Geometry: see drawing. Coordinates: mm, zero at the bounding-box minimum. A direction names the side the tool comes from. Coordinates: 2 decimals unless noted, no trailing zeros. Loops run counter-clockwise (first coordinate to the right, second up) from the corner with the lowest first, then second, coordinate; pieces in that order, holes last. Notation, with made-up numbers: (10, 31) - (63, 31) arc R18 cw to (63, 36) - close; hole circle Ø8 at (28, 56.25). An arc over 180 degrees is marked (long way). Write each question's results on one line, items separated by ' | '. Start each with the question number.
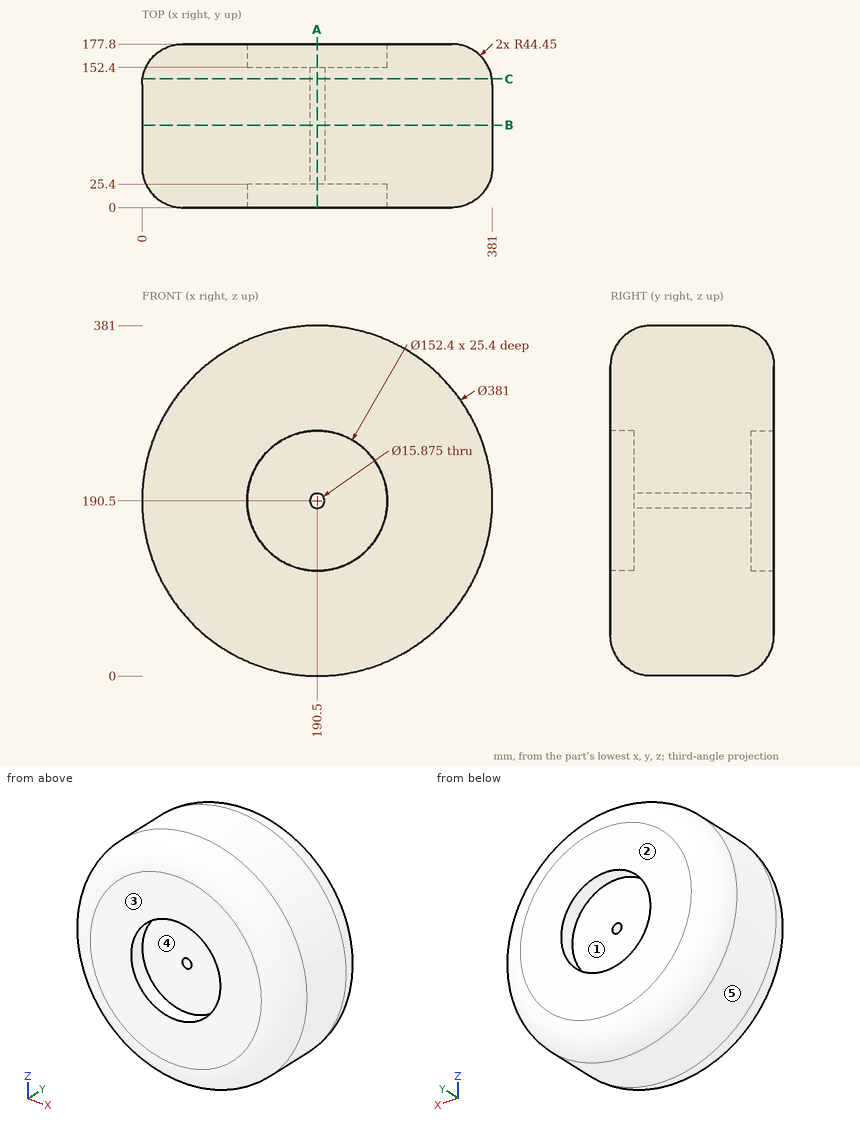
1) Material intervals for line 1 (Z direction, x = 190.5, y = 74); line 2 (X direction, y = 104, z = 190); line 3 (Y direction, x = 140, z = 178.5), sorted ascending. Write a range as [from, to].
2) Section query C-C on y = 140. Output: boundary loops of the cut face in (x, z) (1 decimal).
3) Pull-direction query (Z, two-part tool) for the marked faces 3, 4 and 5; classes: released by +Z, released by -Z, zero draft, split by the parting line, or undercut.
4) Section query A-A on x = 190.5. Output: boundary loops of the cut face in (y, z).
5) Pin query (flat end, axial travel): pin 1 Ø8 at (y, z) = (75, 63) entering from -X; pin 2 Ø12 at (y, z) = (125.5, 145) entering from -X; pin 3 Ø1 at (y, z) = (90.5, 171) entering from +X; pin 4 Ø9.5 at (x, z) = (190.5, 190.5) entering from +Y. Return the tip coordinate at first contact, or that it passes through.
6) Access query for the marked faces 1 and 2. Directions: +Z, -Z, +X, -X, +Y, -Y. A direction counts if a zero-diameter tool reaches every point of the face in a straight line with its end or side. Return the directions, or none.
7) Section query B-B on y = 89.5. Output: boundary loops of the cut face in (x, z) (1 decimal).
Returned:
1) line 1: z = [0, 182.56], [198.44, 381] | line 2: x = [0, 182.58], [198.42, 381] | line 3: y = [25.4, 152.4]
2) outline: circle Ø380 at (190.5, 190.5); hole circle Ø15.9 at (190.5, 190.5)
3) face 3: zero draft | face 4: undercut | face 5: split by the parting line
4) outline: (0, 44.45) arc R44.45 ccw to (44.45, 0) - (133.35, 0) arc R44.45 ccw to (177.8, 44.45) - (177.8, 114.3) - (152.4, 114.3) - (152.4, 182.56) - (25.4, 182.56) - (25.4, 114.3) - (0, 114.3) - close; (0, 266.7) - (25.4, 266.7) - (25.4, 198.44) - (152.4, 198.44) - (152.4, 266.7) - (177.8, 266.7) - (177.8, 336.55) arc R44.45 ccw to (133.35, 381) - (44.45, 381) arc R44.45 ccw to (0, 336.55) - close
5) pin 1: stops at x = 45.46 | pin 2: stops at x = 4.14 | pin 3: stops at x = 380.05 | pin 4: passes through
6) face 1: +Y | face 2: +Z, -Z, +X, -X, +Y
7) outline: circle Ø381 at (190.5, 190.5); hole circle Ø15.9 at (190.5, 190.5)
